from build123d import *

# Parameters (mm, degrees)
BOSS_EXTRUDE1_DEPTH                          = 12.7
SKETCH2_R                                    = 12.827
SKETCH2_R_2                                  = 7.366
CUT_EXTRUDE1_DEPTH                           = 13.7
CBORE_FOR_10_SOCKET_HEAD_CAP_SCREW1_AT_COUNT = 2
CBORE_FOR_10_SOCKET_HEAD_CAP_SCREW1_AT_PITCH = 39.594681461
CBORE_FOR_10_SOCKET_HEAD_CAP_SCREW1_2_COUNT  = 2
CBORE_FOR_10_SOCKET_HEAD_CAP_SCREW1_2_PITCH  = 39.594681461
CBORE_FOR_M3_SHCS1_AT_2_COUNT                = 2
CBORE_FOR_M3_SHCS1_AT_2_PITCH                = 36.769552622
CBORE_FOR_M3_SHCS1_AT_3_COUNT                = 2
CBORE_FOR_M3_SHCS1_AT_3_PITCH                = 26
CBORE_FOR_M3_SHCS1_AT_4_COUNT                = 2
CBORE_FOR_M3_SHCS1_AT_4_PITCH                = 26
FILLET1_R                                    = 1.27
SKETCH13_R                                   = 15.875
SKETCH13_R_2                                 = 12.827
BEARING_POCKET_DEPTH                         = 5.08
SKETCH14_R                                   = 13.97
SKETCH14_R_2                                 = 12.827
CUT_EXTRUDE3_DEPTH                           = 2.667


with BuildPart() as part:
    # Sketch1 → Boss-Extrude1 (new body)
    with BuildSketch(Plane(origin=(0, 0, 0), x_dir=(1, 0, 0), z_dir=(0, 1, 0))):
        with BuildLine():
            Line((-51.110132534, 38.892037987), (4.735019973, 30.109964893))
            ThreePointArc((4.735019973, 30.109964893), (30.48, 0), (4.735019973, -30.109964893))
            Line((4.735019973, -30.109964893), (-51.110132534, -38.892037987))
            ThreePointArc((-51.110132534, -38.892037987), (-96.5962, 0), (-51.110132534, 38.892037987))
        make_face()
    extrude(amount=BOSS_EXTRUDE1_DEPTH)

    # Sketch2 → Cut-Extrude1 (cut, through all)
    with BuildSketch(Plane(origin=(0, 12.7, 0), x_dir=(1, 0, 0), z_dir=(0, 1, 0))):
        with Locations((-57.2262, 0)):
            Circle(SKETCH2_R)
        Circle(SKETCH2_R_2)
    extrude(amount=-CUT_EXTRUDE1_DEPTH, mode=Mode.SUBTRACT)

    # Sketch12 → CBORE for #10 Socket Head Cap Screw1 (revolve, cut)
    with BuildSketch(Plane(origin=(-80.0862, 0, 0), x_dir=(0, 0, -1), z_dir=(1, 0, 0))):
        Polygon((0, 0), (0, 12.7), (2.5527, 12.7), (2.5527, 4.826), (4.7625, 4.826), (4.7625, 0.635), (5.3975, 0), align=None)
    cbore_for_10_socket_head_cap_screw1 = revolve(axis=Axis((-80.0862, -6.35, 0), (0, 1, 0)), mode=Mode.SUBTRACT)

    # CBORE for #10 Socket Head Cap Screw1 at: CBORE for #10 Socket Head Cap Screw1 ×2
    with Locations(*[Vector(0.866025404, 0, -0.5) * (i * CBORE_FOR_10_SOCKET_HEAD_CAP_SCREW1_AT_PITCH) for i in range(1, CBORE_FOR_10_SOCKET_HEAD_CAP_SCREW1_AT_COUNT)]):
        add(cbore_for_10_socket_head_cap_screw1, mode=Mode.SUBTRACT)

    # CBORE for _10 Socket Head Cap Screw1 2: CBORE for #10 Socket Head Cap Screw1 ×2
    with Locations(*[Vector(0.866025404, 0, 0.5) * (i * CBORE_FOR_10_SOCKET_HEAD_CAP_SCREW1_2_PITCH) for i in range(1, CBORE_FOR_10_SOCKET_HEAD_CAP_SCREW1_2_COUNT)]):
        add(cbore_for_10_socket_head_cap_screw1, mode=Mode.SUBTRACT)

    # Sketch16 → CBORE for M3 SHCS1 (revolve, cut)
    with BuildSketch(Plane(origin=(-13, 0, -13), x_dir=(0, 0, -1), z_dir=(1, 0, 0))):
        Polygon((0, 0), (0, 12.7), (1.7, 12.7), (1.7, 3), (3.25, 3), (3.25, 0.75), (4, 0), align=None)
    cbore_for_m3_shcs1 = revolve(axis=Axis((-13, -6.35, -13), (0, 1, 0)), mode=Mode.SUBTRACT)

    # CBORE for M3 SHCS1 at 2: CBORE for M3 SHCS1 ×2
    with Locations(*[Vector(0.707106781, 0, 0.707106781) * (i * CBORE_FOR_M3_SHCS1_AT_2_PITCH) for i in range(1, CBORE_FOR_M3_SHCS1_AT_2_COUNT)]):
        add(cbore_for_m3_shcs1, mode=Mode.SUBTRACT)

    # CBORE for M3 SHCS1 at 3: CBORE for M3 SHCS1 ×2
    with Locations(*[(i * CBORE_FOR_M3_SHCS1_AT_3_PITCH, 0, 0) for i in range(1, CBORE_FOR_M3_SHCS1_AT_3_COUNT)]):
        add(cbore_for_m3_shcs1, mode=Mode.SUBTRACT)

    # CBORE for M3 SHCS1 at 4: CBORE for M3 SHCS1 ×2
    with Locations(*[(0, 0, i * CBORE_FOR_M3_SHCS1_AT_4_PITCH) for i in range(1, CBORE_FOR_M3_SHCS1_AT_4_COUNT)]):
        add(cbore_for_m3_shcs1, mode=Mode.SUBTRACT)

    # Fillet1
    fillet1_edges = [part.edges().sort_by_distance(p)[0] for p in [
        (-7.366, 0, 0),
        (-23.187556281, 0, -34.50100144),
        (30.48, 0, 0),
        (-23.187556281, 0, 34.50100144),
        (-96.5962, 0, 0),
    ]]
    fillet(fillet1_edges, radius=FILLET1_R)

    # Sketch13 → bearing_pocket (cut)
    with BuildSketch(Plane.XZ):
        with Locations((-57.2262, 0)):
            Circle(SKETCH13_R)
        with Locations((-57.2262, 0)):
            Circle(SKETCH13_R_2, mode=Mode.SUBTRACT)
    extrude(amount=-BEARING_POCKET_DEPTH, mode=Mode.SUBTRACT)

    # Sketch14 → Cut-Extrude3 (cut)
    with BuildSketch(Plane(origin=(0, 12.7, 0), x_dir=(1, 0, 0), z_dir=(0, 1, 0))):
        with Locations((-57.2262, 0)):
            Circle(SKETCH14_R)
        with Locations((-57.2262, 0)):
            Circle(SKETCH14_R_2, mode=Mode.SUBTRACT)
    extrude(amount=-CUT_EXTRUDE3_DEPTH, mode=Mode.SUBTRACT)


solid = part.part
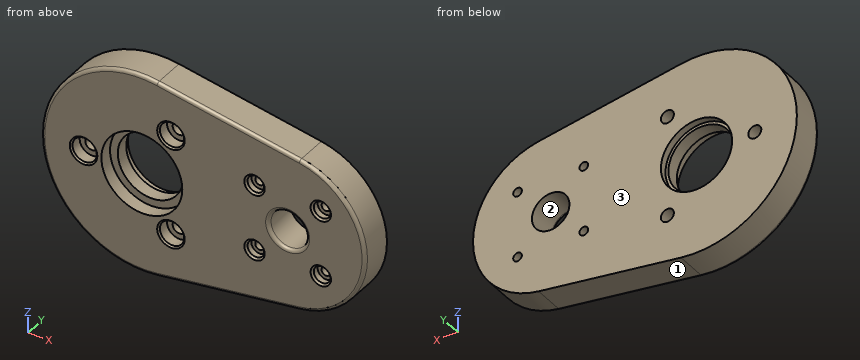
Check sheet for the modelled part. Datum: model origin and axes. Units: mm. Face numbers are marked on the shaded views. Round coordinates to 2 decimals unless told otherwise and drop trailing zeros. One line per item, written item: value.
(1) Release check for a two-part mould opening along X. For the marked faces 1, 2 and 3 record: +X half, -X half, draft (parallel to the pull), parting line (faces both ways), or undercut.
Computed values:
face 1: +X half
face 2: undercut
face 3: draft
(2) Depth check by flat-ended pin: pin 1 Ø5 at (y, z) = (7.5, -11) entering from +X; pin 2 Ø10.5 at (x, z) = (13, -13) entering from +Y; pin 3 Ø3 at (x, z) = (13.5, 14) entering from -Y; pin 4 Ø6 at (y, z) = (3.5, 25) entering from -X. Enter the tip coordinate at first touch or a pass-through.
Computed values:
pin 1: stops at x = 29.27
pin 2: stops at y = 12.7
pin 3: stops at y = 3
pin 4: stops at x = -89.88
(3) Thickness scan on line 1 (X direction, y = 6.4, z = 0); line 2 (X direction, y = 10, z = -13); line 3 (Z direction, x = -58, y = 6.5). Record the ranges inside material, lowest first.
Computed values:
line 1: x = -96.6 to -82.64, -77.53 to -70.05, -44.4 to -7.37, 7.37 to 30.48
line 2: x = -94.39 to -14.7, -11.3 to 11.3, 14.7 to 27.57
line 3: z = -39.36 to -12.8, 12.8 to 39.36
(4) Sectioned sample at A-A, the plane z = 0. Count the separate pieces of the cut face and the enclosed holes in it, then the cut area to 3 significant figures.
Computed values:
separate pieces: 4
enclosed holes: 0
area: 976 mm^2
